Can you work these out from the model? Positions are in its coordinate system, mm. Face numbers are marked on the shaded views. A direction names the side the tool comes from. Give positions to 0.01 mm unless a question says otherwise; leave off trailing zeros. Loops run counter-clockwise (first coordinate to the right, second up) from the corner with the lowest first, then second, coordinate; pieces in that order, holes last.
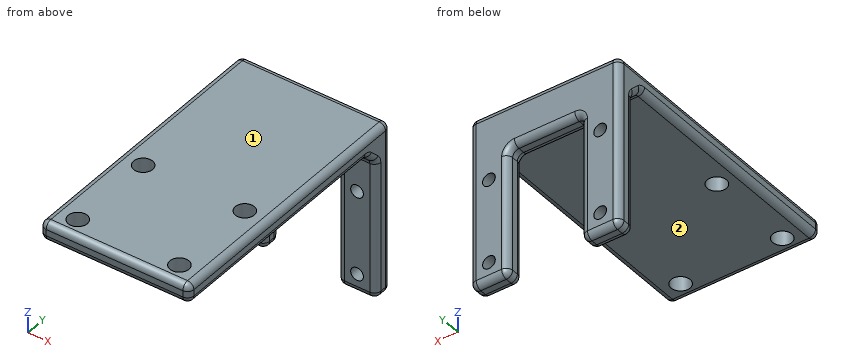
from build123d import *

# Parameters (mm, degrees)
SKETCH_1_W      = 23.5
SKETCH_1_H      = 40
SKETCH_1_R      = 1.5
EXTRUDE_1_DEPTH = 3
SKETCH_2_R      = 1
SKETCH_2_W      = 23.5
SKETCH_2_H      = 3
EXTRUDE_2_DEPTH = 3
CHAMFER_1_SIZE  = 2
FILLET_1_R      = 1


with BuildPart() as part:
    # 草图1 → 凸台-拉伸1 (new body)
    with BuildSketch(Plane.XY):
        Rectangle(SKETCH_1_W, SKETCH_1_H)
        with Locations((-8, -3)):
            Circle(SKETCH_1_R, mode=Mode.SUBTRACT)
        with Locations((8, -3)):
            Circle(SKETCH_1_R, mode=Mode.SUBTRACT)
        with Locations((8, -17)):
            Circle(SKETCH_1_R, mode=Mode.SUBTRACT)
        with Locations((-8, -17)):
            Circle(SKETCH_1_R, mode=Mode.SUBTRACT)
    extrude(amount=EXTRUDE_1_DEPTH)

    # 草图2 → 凸台-拉伸2 (add)
    # profile 1 of 2: a face of its own
    with BuildSketch(Plane(origin=(0, 20, 0), x_dir=(1, 0, 0), z_dir=(0, 1, 0))):
        Polygon((-5.75, 24), (-11.75, 24), (-11.75, 0), (11.75, 0), (11.75, 24), (5.75, 24), (5.75, 4), (-5.75, 4), align=None)
        with Locations(Location((-8.75, 7.8, 0), (0, 0, 270))):
            Circle(SKETCH_2_R, mode=Mode.SUBTRACT)
        with Locations(Location((8.75, 7.8, 0), (0, 0, 270))):
            Circle(SKETCH_2_R, mode=Mode.SUBTRACT)
        with Locations(Location((-8.75, 21, 0), (0, 0, 270))):
            Circle(SKETCH_2_R, mode=Mode.SUBTRACT)
        with Locations(Location((8.75, 21, 0), (0, 0, 270))):
            Circle(SKETCH_2_R, mode=Mode.SUBTRACT)
    # profile 2 of 2: a face of its own
    with BuildSketch(Plane(origin=(0, 20, 0), x_dir=(1, 0, 0), z_dir=(0, 1, 0))):
        with Locations((0, -1.5)):
            Rectangle(SKETCH_2_W, SKETCH_2_H)
    extrude(amount=EXTRUDE_2_DEPTH)

    # 倒角1
    chamfer_1_edges = [part.edges().sort_by_distance(p)[0] for p in [
        (0, 20, 0),
    ]]
    chamfer(chamfer_1_edges, length=CHAMFER_1_SIZE)

    # 圆角1
    fillet_1_edges = [part.edges().sort_by_distance(p)[0] for p in [
        (-11.75, 1.5, 3),
        (0, -20, 3),
        (11.75, 20, -13),
        (-8.75, 20, -24),
        (-5.75, 20, -14),
        (0, 20, -4),
        (8.75, 20, -24),
        (8.75, 23, -24),
        (11.75, 21.5, -24),
        (5.75, 20, -14),
        (5.75, 21.5, -24),
        (0, 23, -4),
        (5.75, 21.5, -4),
        (-5.75, 23, -14),
        (-5.75, 21.5, -4),
        (-8.75, 23, -24),
        (-5.75, 21.5, -24),
        (-11.75, 20, -13),
        (-11.75, 21.5, -24),
        (11.75, 23, -10.5),
        (5.75, 23, -14),
        (-11.75, 23, -10.5),
        (0, 23, 3),
        (11.75, 1.5, 3),
        (0, -20, 0),
        (11.75, -1, 0),
        (0, 20, -2),
        (-11.75, -1, 0),
        (0, 18, 0),
        (-11.75, 19, -1),
        (11.75, 19, -1),
        (11.75, -20, 1.5),
        (-11.75, -20, 1.5),
    ]]
    fillet(fillet_1_edges, radius=FILLET_1_R)


solid = part.part
(1) Will these pins go through, and if not, where does the flat tip stop? P1, Ø1.1, axis at x = -2, y = 21.5, coming from the -Z side; P2, Ø5, axis at x = 8, y = -3, coming from the +Z side; P3, Ø2, axis at x = -5.5, z = -15, coming from the +Y side; P4, Ø3, axis at x = 8.75, z = -7.8, coming from the -Y side.
Returned:
P1: stops at z = -4
P2: stops at z = 3
P3: stops at y = 22.97
P4: stops at y = 20
(2) Which directions (+Z, -Z, +X, -X, +Y, -Y) give clear straight access to the entire face, cutting with the end or side of a thin tool? Please do the marked faces 1 and 2.
Returned:
face 1: +Z, +X, -X, +Y, -Y
face 2: -Z, +X, -X, -Y
(3) Suppose I cut it at C-C on x = 8.75. Give the number of separate pieces and of enclosed holes in the cut face, plus the area to 3 significant figures.
Returned:
separate pieces: 5
enclosed holes: 0
area: 174 mm2
(4) Suppose I cut it at A-A on y = -17. List the corners of the cut face in (x, z) for me.
Returned:
outline: (-11.75, 1) arc R1 ccw to (-10.75, 0) - (-9.5, 0) - (-9.5, 3) - (-10.75, 3) arc R1 ccw to (-11.75, 2) - close; (-6.5, 0) - (6.5, 0) - (6.5, 3) - (-6.5, 3) - close; (9.5, 0) - (10.75, 0) arc R1 ccw to (11.75, 1) - (11.75, 2) arc R1 ccw to (10.75, 3) - (9.5, 3) - close
(5) Suppose I cut it at D-D on y = 16.5. List the corners of the cut face in (x, z) for me.
Returned:
outline: (-11.75, 1) arc R1 ccw to (-10.75, 0) - (10.75, 0) arc R1 ccw to (11.75, 1) - (11.75, 2) arc R1 ccw to (10.75, 3) - (-10.75, 3) arc R1 ccw to (-11.75, 2) - close
(6) Suppose I cut it at B-B on z = -9.75. List the corners of the cut face in (x, y) for me, plus the area to 3 significant figures.
Returned:
outline: (-11.75, 21) arc R1 ccw to (-10.75, 20) - (-6.75, 20) arc R1 ccw to (-5.75, 21) - (-5.75, 22) arc R1 ccw to (-6.75, 23) - (-10.75, 23) arc R1 ccw to (-11.75, 22) - close; (5.75, 21) arc R1 ccw to (6.75, 20) - (10.75, 20) arc R1 ccw to (11.75, 21) - (11.75, 22) arc R1 ccw to (10.75, 23) - (6.75, 23) arc R1 ccw to (5.75, 22) - close
area: 34.3 mm2
(7) Please list where these lines run through material, in increasing order: probe 1 along Y at (x, z) = (-8, 2); probe 2 along X at (y, z) = (20.95, -21).
Returned:
probe 1: y = -20 to -18.5, -15.5 to -4.5, -1.5 to 23
probe 2: x = -11.75 to -9.75, -7.75 to -5.75, 5.75 to 7.75, 9.75 to 11.75
